```python
from build123d import *

# Parameters (mm, degrees)
CUT_EXTRUDE2_DEPTH = 14.2748


with BuildPart() as part:
    # Sketch3 → Revolve1 (revolve)
    with BuildSketch(Plane.XY):
        with BuildLine():
            Line((4.699, 4.9911), (4.699, 0.9525))
            Line((4.699, 0.9525), (3.7465, 0))
            Line((3.7465, 0), (0, 0))
            Line((0, 0), (0, 14.2748))
            ThreePointArc((0, 14.2748), (5.586411751, 13.779471711), (10.9985175, 12.308941969))
            Line((10.9985175, 12.308941969), (10.9985175, 7.9248))
            Line((10.9985175, 7.9248), (4.1275, 7.9248))
            ThreePointArc((4.1275, 7.9248), (3.858092316, 7.813207684), (3.7465, 7.5438))
            Line((3.7465, 7.5438), (3.7465, 5.9436))
            Line((3.7465, 5.9436), (4.699, 4.9911))
        make_face()
    revolve(axis=Axis((0, -1000, 0), (0, 1, 0)))

    # Sketch1 → Cut-Extrude2 (cut)
    with BuildSketch(Plane(origin=(0, 0, 0), x_dir=(1, 0, 0), z_dir=(0, 1, 0))):
        with BuildLine():
            ThreePointArc((-5.499261314, -9.525), (0, -10.998522628), (5.499261314, -9.525))
            Line((5.499261314, -9.525), (-5.499261314, -9.525))
        make_face()
        with BuildLine():
            ThreePointArc((-10.998522628, 0), (-9.525, -5.499261314), (-5.499261314, -9.525))
            Line((-5.499261314, -9.525), (-10.998522628, 0))
        make_face()
        with BuildLine():
            ThreePointArc((5.499261314, -9.525), (9.525, -5.499261314), (10.998522628, 0))
            Line((10.998522628, 0), (5.499261314, -9.525))
        make_face()
        with BuildLine():
            Line((5.499261314, 9.525), (10.998522628, 0))
            ThreePointArc((10.998522628, 0), (9.525, 5.499261314), (5.499261314, 9.525))
        make_face()
        with BuildLine():
            Line((-5.499261314, 9.525), (5.499261314, 9.525))
            ThreePointArc((5.499261314, 9.525), (0, 10.998522628), (-5.499261314, 9.525))
        make_face()
        with BuildLine():
            Line((-10.998522628, 0), (-5.499261314, 9.525))
            ThreePointArc((-5.499261314, 9.525), (-9.525, 5.499261314), (-10.998522628, 0))
        make_face()
    extrude(amount=CUT_EXTRUDE2_DEPTH, mode=Mode.SUBTRACT)


solid = part.part
```
The listing builds one solid part. Answer for the finished solid, in the listing's coordinates (mm). A direction names the side the tool comes from. Give positions to 0.01 mm unless a question says otherwise; leave off trailing zeros. Write each loop counter-clockwise with the first axis right and the second up, starting at its lowest first coordinate (ties: lowest second). Pieces come first, ordered by that corner, then holes. Notation, with made-up numbers: (24, -26) -> (54, -26) arc R31 ccw to (54, 2) -> close; hole circle Ø6 at (-1.75, 71.25). An arc over 180 degrees is marked (long way). Write item = value, one per line. Start each with the question number.
1) The part is cut by section C-C, the plane y = 6.5. Determine the outline of the cut face in (x, z).
2) The part is cut by section D-D, the plane z = -6.25. Determine the outline of the cut face in (x, y).
3) Straight lines are drawn through the part: line 1 along Y through (x, z) = (-4.5, 0.25); line 2 along X through (y, z) = (9, -7.25); line 3 along Y through (x, z) = (-5, 1.25). For each, find the intervals that lie inside material, in ascending order.
4) Which of the six approach directions +Z, -Z, +X, -X, +Y, -Y give full straight-line access (tool end or side, diameter ignored) to faces 1 (the face through (8.287, 10.334, 4.696)), 2 (the face through (-0.488, 6.732, -3.715)), 3 (the face through (-0.61, 2.94, -4.66))?
5) Each of these flat-tipped pins is pushed along its axis until it touches: pin 1 (3 mm diameter, centred on y = 8.5, z = -6, fed in from -X); pin 2 (1.5 mm diameter, centred on y = 4.5, z = 3.5, fed in from -X); pin 3 (8 mm diameter, centred on y = 12, z = 6.5, fed in from +X); pin 4 (5 mm diameter, centred on y = 11, z = -1.5, fed in from +X). Where does it stop, or does it pass through?
Solutions:
q1.outline = circle Ø7.49 at (0, 0)
q2.outline = (-7.39, 7.92) -> (7.39, 7.92) -> (7.39, 12.76) arc R31.13 ccw to (-7.39, 12.76) -> close
q3.line_1 = 0.76 to 5.18, 7.92 to 13.95
q3.line_2 = -6.81 to 6.81
q3.line_3 = 7.92 to 13.85
q4.face_1 = +Z, +X, +Y, -Y
q4.face_2 = none
q4.face_3 = -Y
q5.pin_1 = -8.4
q5.pin_2 = -3.81
q5.pin_3 = 9.56
q5.pin_4 = 11
